The model under review builds one solid part; all positions refer to its coordinate system, in mm. A direction names the side the tool comes from. Give positions to 0.01 mm unless a question says otherwise; leave off trailing zeros. Answer as a JSON object with one key per item and string values.
from build123d import *

# Parameters (mm, degrees)
RESSALTO_EXTRUS_O1_DEPTH = 4
ESBO_O8_OUTSIDE_W        = 77.722
ESBO_O8_OUTSIDE_H        = 57.722
ESBO_O8_OUTSIDE_R        = 0.9
CORTE_EXTRUS_O8_DEPTH    = 5
FILETE4_R                = 4
ESBO_O11_W               = 53
ESBO_O11_H               = 33
RESSALTO_EXTRUS_O4_DEPTH = 1
CORTE_EXTRUS_O9_START    = -2
ESBO_O3_OUTSIDE_W        = 77.734
ESBO_O3_OUTSIDE_H        = 57.734
CORTE_EXTRUS_O9_DEPTH    = 8
RESSALTO_EXTRUS_O5_DEPTH = 3
FILETE5_R                = 1
FILETE6_R                = 1


with BuildPart() as part:
    # Esboço1 → Ressalto-extrusão1 (new body)
    with BuildSketch(Plane.XY):
        with BuildLine():
            Line((4, 0), (57, 0))
            ThreePointArc((57, 0), (59.828427125, -1.171572875), (61, -4))
            Line((61, -4), (61, -37))
            ThreePointArc((61, -37), (59.828427125, -39.828427125), (57, -41))
            Line((57, -41), (4, -41))
            ThreePointArc((4, -41), (1.171572875, -39.828427125), (0, -37))
            Line((0, -37), (0, -4))
            ThreePointArc((0, -4), (1.171572875, -1.171572875), (4, 0))
        make_face()
    extrude(amount=RESSALTO_EXTRUS_O1_DEPTH)

    # Esboço8 outside → Corte-extrusão8 (cut)
    # profile 1 of 7: a face of its own
    with BuildSketch(Plane.XY.offset(4)):
        with Locations((30.5, -20.5)):
            Rectangle(ESBO_O8_OUTSIDE_W, ESBO_O8_OUTSIDE_H)
        with BuildLine():
            Line((0, -4), (0, -37))
            ThreePointArc((0, -37), (1.171572875, -39.828427125), (4, -41))
            Line((4, -41), (57, -41))
            ThreePointArc((57, -41), (59.828427125, -39.828427125), (61, -37))
            Line((61, -37), (61, -4))
            ThreePointArc((61, -4), (59.828427125, -1.171572875), (57, 0))
            Line((57, 0), (4, 0))
            ThreePointArc((4, 0), (1.171572875, -1.171572875), (0, -4))
        make_face(mode=Mode.SUBTRACT)
    # profile 2 of 7: a face of its own
    with BuildSketch(Plane.XY.offset(4)):
        with Locations((46.84, -18.41)):
            Circle(ESBO_O8_OUTSIDE_R)
    # profile 3 of 7: a face of its own
    with BuildSketch(Plane.XY.offset(4)):
        with Locations((48.84, -18.41)):
            Circle(ESBO_O8_OUTSIDE_R)
    # profile 4 of 7: a face of its own
    with BuildSketch(Plane.XY.offset(4)):
        with Locations((50.84, -18.41)):
            Circle(ESBO_O8_OUTSIDE_R)
    # profile 5 of 7: a face of its own
    with BuildSketch(Plane.XY.offset(4)):
        with Locations((52.84, -18.41)):
            Circle(ESBO_O8_OUTSIDE_R)
    # profile 6 of 7: a face of its own
    with BuildSketch(Plane.XY.offset(4)):
        with BuildLine():
            Line((34.2277501, -19.41), (42.0522499, -19.41))
            ThreePointArc((42.0522499, -19.41), (42.550015401, -19.046408603), (42.74, -18.46))
            Line((42.74, -18.46), (42.74, -17.11))
            ThreePointArc((42.74, -17.11), (42.447106781, -16.402893219), (41.74, -16.11))
            Line((41.74, -16.11), (34.54, -16.11))
            ThreePointArc((34.54, -16.11), (33.832893219, -16.402893219), (33.54, -17.11))
            Line((33.54, -17.11), (33.54, -18.46))
            ThreePointArc((33.54, -18.46), (33.729984599, -19.046408603), (34.2277501, -19.41))
        make_face()
    # profile 7 of 7: a face of its own
    with BuildSketch(Plane.XY.offset(4)):
        with BuildLine():
            Line((32.84, -22.76), (32.84, -28.46))
            ThreePointArc((32.84, -28.46), (33.015735931, -28.884264069), (33.44, -29.06))
            Line((33.44, -29.06), (46.64, -29.06))
            ThreePointArc((46.64, -29.06), (47.064264069, -28.884264069), (47.24, -28.46))
            Line((47.24, -28.46), (47.24, -22.76))
            ThreePointArc((47.24, -22.76), (47.064264069, -22.335735931), (46.64, -22.16))
            Line((46.64, -22.16), (33.44, -22.16))
            ThreePointArc((33.44, -22.16), (33.015735931, -22.335735931), (32.84, -22.76))
        make_face()
    extrude(amount=-CORTE_EXTRUS_O8_DEPTH, mode=Mode.SUBTRACT)

    # Filete4
    filete4_edges = [part.edges().sort_by_distance(p)[0] for p in [
        (1.171572875, -1.171572875, 4),
        (0, -20.5, 4),
        (1.171572875, -39.828427125, 4),
        (30.5, -41, 4),
        (59.828427125, -39.828427125, 4),
        (61, -20.5, 4),
        (59.828427125, -1.171572875, 4),
        (30.5, 0, 4),
    ]]
    fillet(filete4_edges, radius=FILETE4_R - 0.0001)  # a hair under: the kernel refuses the full size

    # Esboço11 → Ressalto-extrusão4 (add)
    with BuildSketch(Plane(origin=(0, 0, 0), x_dir=(-1, 0, 0), z_dir=(0, 0, -1))):
        with Locations((-30.5, -20.5)):
            Rectangle(ESBO_O11_W, ESBO_O11_H)
    extrude(amount=RESSALTO_EXTRUS_O4_DEPTH)

    # Esboço3 outside → Corte-extrusão9 (cut)
    # profile 1 of 3: a face of its own
    with BuildSketch(Plane.XY.offset(4).offset(CORTE_EXTRUS_O9_START)):
        with Locations((30.5, -20.5)):
            Rectangle(ESBO_O3_OUTSIDE_W, ESBO_O3_OUTSIDE_H)
        with BuildLine():
            Line((0, -4), (0, -37))
            ThreePointArc((0, -37), (1.171572875, -39.828427125), (4, -41))
            Line((4, -41), (57, -41))
            ThreePointArc((57, -41), (59.828427125, -39.828427125), (61, -37))
            Line((61, -37), (61, -4))
            ThreePointArc((61, -4), (59.828427125, -1.171572875), (57, 0))
            Line((57, 0), (4, 0))
            ThreePointArc((4, 0), (1.171572875, -1.171572875), (0, -4))
        make_face(mode=Mode.SUBTRACT)
    # profile 2 of 3: a face of its own
    with BuildSketch(Plane.XY.offset(4).offset(CORTE_EXTRUS_O9_START)):
        with BuildLine():
            Line((53.69, -18.41), (53.69, -19.41))
            Line((53.69, -19.41), (56.34, -19.41))
            Line((56.34, -19.41), (56.34, -21.01))
            Line((56.34, -21.01), (30.24, -21.01))
            Line((30.24, -21.01), (30.24, -19.41))
            Line((30.24, -19.41), (34.2277501, -19.41))
            ThreePointArc((34.2277501, -19.41), (33.729984599, -19.046408603), (33.54, -18.46))
            Line((33.54, -18.46), (33.54, -17.11))
            ThreePointArc((33.54, -17.11), (33.832893219, -16.402893219), (34.54, -16.11))
            Line((34.54, -16.11), (41.74, -16.11))
            ThreePointArc((41.74, -16.11), (42.447106781, -16.402893219), (42.74, -17.11))
            Line((42.74, -17.11), (42.74, -18.46))
            ThreePointArc((42.74, -18.46), (42.550015401, -19.046408603), (42.0522499, -19.41))
            Line((42.0522499, -19.41), (43.99, -19.41))
            Line((43.99, -19.41), (43.99, -18.41))
            ThreePointArc((43.99, -18.41), (44.68752686, -17.573787143), (45.635298686, -18.11))
            Line((45.635298686, -18.11), (46.044701314, -18.11))
            ThreePointArc((46.044701314, -18.11), (46.84, -17.56), (47.635298686, -18.11))
            Line((47.635298686, -18.11), (48.044701314, -18.11))
            ThreePointArc((48.044701314, -18.11), (48.84, -17.56), (49.635298686, -18.11))
            Line((49.635298686, -18.11), (50.044701314, -18.11))
            ThreePointArc((50.044701314, -18.11), (50.84, -17.56), (51.635298686, -18.11))
            Line((51.635298686, -18.11), (52.044701314, -18.11))
            ThreePointArc((52.044701314, -18.11), (52.99247314, -17.573787143), (53.69, -18.41))
        make_face()
    # profile 3 of 3: a face of its own
    with BuildSketch(Plane.XY.offset(4).offset(CORTE_EXTRUS_O9_START)):
        with BuildLine():
            Line((33.44, -22.16), (46.64, -22.16))
            ThreePointArc((46.64, -22.16), (47.064264069, -22.335735931), (47.24, -22.76))
            Line((47.24, -22.76), (47.24, -28.46))
            ThreePointArc((47.24, -28.46), (47.064264069, -28.884264069), (46.64, -29.06))
            Line((46.64, -29.06), (33.44, -29.06))
            ThreePointArc((33.44, -29.06), (33.015735931, -28.884264069), (32.84, -28.46))
            Line((32.84, -28.46), (32.84, -22.76))
            ThreePointArc((32.84, -22.76), (33.015735931, -22.335735931), (33.44, -22.16))
        make_face()
    extrude(amount=-CORTE_EXTRUS_O9_DEPTH, mode=Mode.SUBTRACT)

    # Esboço13 → Ressalto-extrusão5 (add)
    with BuildSketch(Plane(origin=(0, 0, -1), x_dir=(-1, 0, 0), z_dir=(0, 0, -1))):
        Polygon((-57, -4), (-4, -4), (-4, -37), (-57, -37), (-57, -25), (-55, -25), (-55, -35), (-6, -35), (-6, -6), (-55, -6), (-55, -15.992966124), (-57, -15.992966124), align=None)
    extrude(amount=RESSALTO_EXTRUS_O5_DEPTH)

    # Filete5
    filete5_edges = [part.edges().sort_by_distance(p)[0] for p in [
        (56, -15.992966124, -4),
    ]]
    fillet(filete5_edges, radius=FILETE5_R)

    # Filete6
    filete6_edges = [part.edges().sort_by_distance(p)[0] for p in [
        (56, -25, -4),
    ]]
    fillet(filete6_edges, radius=FILETE6_R)


solid = part.part
Q1. To check wall thickness, follow probe 1 along Y at (x, z) = (45, -0.75); probe 2 along X at (y, z) = (-18.41, 3.1); probe 3 along Y at (x, z) = (7.5, -3). State the ranges of each line that lie inside material, in increasing order. Write a range as [from, to].
Results:
{"probe 1": "y = [-37, -29.06], [-22.16, -21.01], [-17.58, -4]", "probe 2": "x = [1.47, 33.54], [42.74, 45.94], [47.74, 47.94], [49.74, 49.94], [51.74, 51.94], [53.74, 59.53]", "probe 3": "y = [-37, -35], [-6, -4]"}
Q2. For faces 5 (the face through (43, -19.41, 1)), 6 (the face through (48.72, -17.52, 2.47)), 7 (the face through (47.24, -26, 2)), list the 3-axis set-ups (+Z, -Z, +X, -X, +Y, -Y) from which the entire face can be reached by the end or side of a thin tool; tool diameter is ignored.
Results:
{"face 5": "-Z", "face 6": "+Z", "face 7": "+Z, -Z"}
Q3. The part is to be moulded in two halves that separate along X. For faces 1 (the face through (6, -21, -2)), 2 (the face through (38, -19.41, 3)), 3 (the face through (1.141, -20.269, 2.797)), 4 (the face through (30.871, -1.141, 2.797)), say which applies: +X half, -X half, draft (parallel to the pull), parting line (faces both ways), or undercut.
Results:
{"face 1": "undercut", "face 2": "undercut", "face 3": "-X half", "face 4": "draft"}
Q4. Consider section A-A, the plane x = 40.5. State how many separate pieces and enclosed holes the cut face has, plus the area to 3 significant figures.
Results:
{"separate pieces": "3", "enclosed holes": "0", "area": "146 mm^2"}
Q5. Clearance check with flat-ended pins moving along their axes: pin 1 Ø8.5 at (x, y) = (22, -16.5) entering from -Z; pin 2 Ø3 at (y, z) = (-25, 2) entering from -X; pin 3 Ø1.2 at (y, z) = (-24, -2.5) entering from +X. State where each tip first meets the part, or that it passes through.
Results:
{"pin 1": "stops at z = -1", "pin 2": "stops at x = 0.03", "pin 3": "stops at x = 6"}
